```python
from build123d import *

# Parameters (mm, degrees)
F0_R     = 6.35
F0_R_2   = 11
F1_DEPTH = 4.8


with BuildPart() as f1:
    # F0 (on Top) → F1 (new body)
    with BuildSketch(Plane.XY):
        with BuildLine():
            ThreePointArc((0, -14.5), (10.2530483272, -10.2530483272), (14.5, 0))
            ThreePointArc((14.5, 0), (14.0059244812, 3.752876154), (12.5573683549, 7.25))
            ThreePointArc((12.5573683549, 7.25), (0, 14.5), (-12.5573683549, 7.25))
            ThreePointArc((-12.5573683549, 7.25), (-12.5573683549, -7.25), (0, -14.5))
        make_face()
        Circle(F0_R, mode=Mode.SUBTRACT)
        with BuildLine():
            ThreePointArc((12.5573683549, 7.25), (14.0059244812, 3.752876154), (14.5, 0))
            ThreePointArc((14.5, 0), (10.2530483272, -10.2530483272), (0, -14.5))
            ThreePointArc((0, -14.5), (7.25, -16.4426316451), (12.5573683549, -21.75))
            ThreePointArc((12.5573683549, -21.75), (37.6721050646, -21.75), (25.1147367097, 0))
            ThreePointArc((25.1147367097, 0), (17.8647367097, 1.9426316451), (12.5573683549, 7.25))
        make_face()
        with Locations((25.1147367097, -14.5)):
            Circle(F0_R_2, mode=Mode.SUBTRACT)
        with BuildLine():
            ThreePointArc((-12.5573683549, 7.25), (0, 14.5), (12.5573683549, 7.25))
            ThreePointArc((12.5573683549, 7.25), (10.6147367097, 14.5), (12.5573683549, 21.75))
            ThreePointArc((12.5573683549, 21.75), (0, 43.5), (-12.5573683549, 21.75))
            ThreePointArc((-12.5573683549, 21.75), (-10.6147367097, 14.5), (-12.5573683549, 7.25))
        make_face()
        with Locations((0, 29)):
            Circle(F0_R_2, mode=Mode.SUBTRACT)
        with BuildLine():
            ThreePointArc((-12.5573683549, -21.75), (-7.25, -16.4426316451), (0, -14.5))
            ThreePointArc((0, -14.5), (-12.5573683549, -7.25), (-12.5573683549, 7.25))
            ThreePointArc((-12.5573683549, 7.25), (-17.8647367097, 1.9426316451), (-25.1147367097, 0))
            ThreePointArc((-25.1147367097, 0), (-37.6721050646, -21.75), (-12.5573683549, -21.75))
        make_face()
        with Locations((-25.1147367097, -14.5)):
            Circle(F0_R_2, mode=Mode.SUBTRACT)
    extrude(amount=F1_DEPTH)


solid = f1.part
```
Geometry check sheet. Reference: the model listing, model coordinates, mm. Coordinates: 2 decimals unless noted, no trailing zeros. Write each loop counter-clockwise with the first axis right and the second up, starting at its lowest first coordinate (ties: lowest second). Pieces come first, ordered by that corner, then holes. Notation, with made-up numbers: M -6.5,61 L 52.5,61 A18 ccw 52.5,73 Z; hole C -24,13 d2. An arc over 180 degrees is marked long. One line per item, written item: value. Start each with the question number.
(1) Sectioned sample at D-D, the plane y = -9. Enter the section's corners in (x, z).
(2) Sectioned sample at C-C, the plane x = 27. Enter the section's corners in (y, z).
(3) Scan lines: line 1 along Y through (x, z) = (0, 2.5); line 2 along Y through (x, z) = (-3.5, 2.85); line 3 along X through (y, z) = (-11.5, 3.4). Record each from-to range of solid material in increasing order. Write a range as [from, to].
(4) Depth check by flat-ended pin: pin 1 (20 mm diameter, centred on x = 25.11, y = -14.5, fed in from +Z); pin 2 (2 mm diameter, centred on y = 24.5, z = 1.5, fed in from -X); pin 3 (2 mm diameter, centred on y = 21, z = 2.5, fed in from +X); pin 4 (1.5 mm diameter, centred on y = 11, z = 2, fed in from +X). Enter the tip coordinate at first touch or a pass-through.
(5) Release check for a two-part mould opening along Y. For faces 1 (the face through (0, 7, 0)), 2 (the face through (-2.38, 18.26, 2.37)), 3 (the face through (-27.5, -25.24, 2.37)) record: released by +Y, released by -Y, zero draft, split by the parting line, or undercut.
(6) Sectioned sample at A-A, the plane y = 29. Enter the section's corners in (x, z).
(7) Sectioned sample at B-B, the plane z = 0.75. Enter the section's corners in (x, y), and give its area (3 significant figures).
Filled sheet:
1. outline: M -38.53,0 L -34.64,0 L -34.64,4.8 L -38.53,4.8 Z; M -15.59,0 L 15.59,0 L 15.59,4.8 L -15.59,4.8 Z; M 34.64,0 L 38.53,0 L 38.53,4.8 L 34.64,4.8 Z
2. outline: M -28.88,0 L -25.34,0 L -25.34,4.8 L -28.88,4.8 Z; M -3.66,0 L -0.12,0 L -0.12,4.8 L -3.66,4.8 Z
3. line 1: [-14.5, -6.35], [6.35, 18], [40, 43.5]
3. line 2: [-14.93, -5.3], [5.3, 18.57], [39.43, 43.07]
3. line 3: [-39.3, -35.7], [-14.53, 14.53], [35.7, 39.3]
4. pin 1: through
4. pin 2: x = -14.07
4. pin 3: x = 12.7
4. pin 4: x = 11.25
5. face 1: zero draft
5. face 2: undercut
5. face 3: undercut
6. outline: M -14.5,0 L -11,0 L -11,4.8 L -14.5,4.8 Z; M 11,0 L 14.5,0 L 14.5,4.8 L 11,4.8 Z
7. outline: M -25.11,0 A14.5 ccw long -12.56,-21.75 A14.5 cw 12.56,-21.75 A14.5 ccw long 25.11,0 A14.5 cw 12.56,21.75 A14.5 ccw long -12.56,21.75 A14.5 cw Z; hole C -25.11,-14.5 d22; hole C 0,29 d22; hole C 0,0 d12.7; hole C 25.11,-14.5 d22
7. area: 1,580 mm²
